Verification items for the finished model (mm, model axes). A direction names the side the tool comes from. Coordinates: 2 decimals unless noted, no trailing zeros. Order: outer loops, then holes, each group sorted by start corner. A loop starts at its lowest first (then second) coordinate and runs counter-clockwise, first axis right, second up. Notation, with made-up numbers: (77, 71) -> (102, 71) arc R27 cw to (102, 87) -> close; hole circle Ø2 at (-25, 87.25). An arc over 180 degrees is marked (long way). Answer as CSV lines item,"result".
```python
from build123d import *

# Parameters (mm, degrees)
SKETCH_1_R               = 2.45
EXTRUDE_1_DEPTH          = 15
CUT_EXTRUDE_1_DEPTH      = 16.39496671
CUT_EXTRUDE_1_DEPTH_BACK = 16.39496671
SKETCH_3_R               = 1.25
EXTRUDE_2_DEPTH          = 5
FILLET_1_R               = 0.3
FILLET_2_R               = 0.2


with BuildPart() as part:
    # 스케치1 → 보스-돌출1 (new body)
    with BuildSketch(Plane.XY):
        Circle(SKETCH_1_R)
    extrude(amount=EXTRUDE_1_DEPTH)

    # 스케치2 → 컷-돌출1 (cut, two sides: drawn at the far end of the back side and taken through both)
    with BuildSketch(Plane(origin=(0, 0, 0), x_dir=(1, 0, 0), z_dir=(0, 1, 0)).offset(-CUT_EXTRUDE_1_DEPTH_BACK)):
        with BuildLine():
            Line((-4.45, -6.5), (-4.45, -10.5))
            ThreePointArc((-4.45, -10.5), (-2.45, -12.5), (-0.45, -10.5))
            Line((-0.45, -10.5), (-0.45, -6.5))
            ThreePointArc((-0.45, -6.5), (-2.45, -4.5), (-4.45, -6.5))
        make_face()
    extrude(amount=CUT_EXTRUDE_1_DEPTH + CUT_EXTRUDE_1_DEPTH_BACK, mode=Mode.SUBTRACT)

    # 스케치3 → 보스-돌출2 (add)
    with BuildSketch(Plane.XY.offset(15)):
        Circle(SKETCH_3_R)
    extrude(amount=EXTRUDE_2_DEPTH)

    # 필렛1
    fillet_1_edges = [part.edges().sort_by_distance(p)[0] for p in [
        (-2.45, 0, 0),
    ]]
    fillet(fillet_1_edges, radius=FILLET_1_R)

    # 필렛2
    fillet_2_edges = [part.edges().sort_by_distance(p)[0] for p in [
        (-1.25, 0, 15),
    ]]
    fillet(fillet_2_edges, radius=FILLET_2_R)


solid = part.part
```
Item 1: Section check A-A, the plane y = 0. Record the boundary of the cut face in (x, z), plus the area to 3 significant figures.
Answer list:
outline,"(-2.45, 0.3) arc R0.3 ccw to (-2.15, 0) -> (2.15, 0) arc R0.3 ccw to (2.45, 0.3) -> (2.45, 15) -> (1.45, 15) arc R0.2 cw to (1.25, 15.2) -> (1.25, 20) -> (-1.25, 20) -> (-1.25, 15.2) arc R0.2 cw to (-1.45, 15) -> (-2.45, 15) -> (-2.45, 12.5) arc R2 cw to (-0.45, 10.5) -> (-0.45, 6.5) arc R2 cw to (-2.45, 4.5) -> close"
area,"71.7 mm2"
Item 2: Tool access check on faces 1 (the flat face through (0, -2, 15)), 2 (the cylindrical face through (-0.824, -0.034, 11.665)), 3 (the cylindrical face through (2.337, 0.736, 7.547)). Record the directions out of +Z, -Z, +X, -X, +Y, -Y that give a thin tool (end or side, any length) a straight path to the whole face; none if there is none.
Answer list:
face 1,"+Z"
face 2,"-X, +Y, -Y"
face 3,"+Z, -Z"
Item 3: Section check B-B, the plane x = 0. Record the boundary of the cut face in (y, z), plus the area to 3 significant figures.
Answer list:
outline,"(-2.45, 0.3) arc R0.3 ccw to (-2.15, 0) -> (2.15, 0) arc R0.3 ccw to (2.45, 0.3) -> (2.45, 15) -> (1.45, 15) arc R0.2 cw to (1.25, 15.2) -> (1.25, 20) -> (-1.25, 20) -> (-1.25, 15.2) arc R0.2 cw to (-1.45, 15) -> (-2.45, 15) -> close"
area,"86.0 mm2"
Item 4: Section check C-C, the plane z = 10. Record the boundary of the cut face in (x, y).
Answer list:
outline,"(-0.45, -2.41) arc R2.45 ccw (long way) to (-0.45, 2.41) -> close"
Item 5: Thickness scan on line 1 (Z direction, x = 1.95, y = -0.8); line 2 (Z direction, x = -1.1, y = -0.25); line 3 (Z direction, x = -1.5, y = -1.2). Record the ranges inside material, lowest first.
Answer list:
line 1,"0 to 15"
line 2,"0 to 5.02, 11.98 to 20"
line 3,"0 to 4.74, 12.26 to 15"
Item 6: Release check for a two-part mould opening along Z. For faces 4 (the flat face through (0, 0, 20)), 5 (the cylindrical face through (-0.8, -0.03, 5.37)), 6 (the flat face through (0, 0, 0)) record: +Z half, -Z half, draft (parallel to the pull), parting line (faces both ways), or undercut.
Answer list:
face 4,"+Z half"
face 5,"undercut"
face 6,"-Z half"
Item 7: Section check D-D, the plane z = 15.75. Record the boundary of the cut face in (x, y), plus the area to 3 significant figures.
Answer list:
outline,"circle Ø2.5 at (0, 0)"
area,"4.91 mm2"
